Model file for the job. Use its own axes, mm. Face numbers are marked on the shaded views. A direction names the side the tool comes from. Round coordinates to 2 decimals unless told otherwise and drop trailing zeros. Loops run counter-clockwise (first coordinate to the right, second up) from the corner with the lowest first, then second, coordinate; pieces in that order, holes last. Notation, with made-up numbers: M -21.75,59 L -3.75,59 A23 ccw -3.75,84 Z; hole C -31,80 d4. An arc over 180 degrees is marked long. Use a Markdown table: item, result. Add a question column.
Q1. Tool access for the marked faces 1 and 2: list every direction of +Z, -Z, +X, -X, +Y, -Y with a clear straight run to the whole face (end or side of a thin tool).
Q2. Pin check, flat tips, straight feed: pin 1 (1 mm diameter, centred on y = 85.5, z = -4, fed in from -X); pin 2 (6 mm diameter, centred on x = 1, z = -2.5, fed in from -Y); pin 3 (1.5 mm diameter, centred on x = 14, y = 87.5, fed in from +Z); pin 4 (5 mm diameter, centred on x = -5, y = 43, fed in from -Z). Stop position of each tip, or through.
Q3. Cut at B-B (z = 0). Give the cut face in (x, y).
Q4. Cut at C-C (y = 109.5). Give the cut face in (x, z), plus the area to 3 significant figures.
Q5. Probe line 1 (Y direction, x = 8, z = 9); line 2 (X direction, y = 116, z = 1); line 3 (X direction, y = 85.5, z = 6.5). List the from-to ranges inside material, lowest first. Write a range as from..to.
Q6. Cut at A-A (x = 0). Give the cut face in (y, z), plus the area to 3 significant figures.
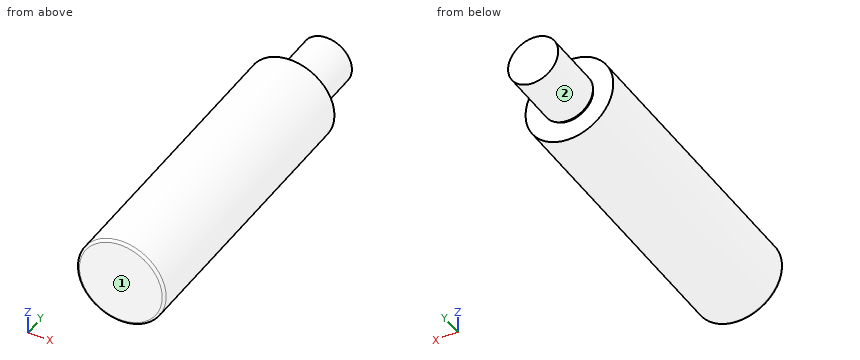
from build123d import *

# Parameters (mm, degrees)
SKETCH1_R           = 17.5
BOSS_EXTRUDE1_DEPTH = 142
SKETCH2_OUTSIDE_W   = 67.076
SKETCH2_OUTSIDE_H   = 67.076
SKETCH2_OUTSIDE_R   = 10
CUT_EXTRUDE1_DEPTH  = 25
SKETCH3_OUTSIDE_W   = 67.076
SKETCH3_OUTSIDE_H   = 67.076
SKETCH3_OUTSIDE_R   = 9.5
CUT_EXTRUDE2_DEPTH  = 1
FILLET1_R           = 1


with BuildPart() as part:
    # Sketch1 → Boss-Extrude1 (new body)
    with BuildSketch(Plane(origin=(0, 0, 0), x_dir=(1, 0, 0), z_dir=(0, 1, 0))):
        Circle(SKETCH1_R)
    extrude(amount=BOSS_EXTRUDE1_DEPTH)

    # Sketch2 outside → Cut-Extrude1 (cut)
    with BuildSketch(Plane(origin=(0, 142, 0), x_dir=(1, 0, 0), z_dir=(0, 1, 0))):
        Rectangle(SKETCH2_OUTSIDE_W, SKETCH2_OUTSIDE_H)
        Circle(SKETCH2_OUTSIDE_R, mode=Mode.SUBTRACT)
    extrude(amount=-CUT_EXTRUDE1_DEPTH, mode=Mode.SUBTRACT)

    # Sketch3 outside → Cut-Extrude2 (cut)
    with BuildSketch(Plane(origin=(0, 117, 0), x_dir=(1, 0, 0), z_dir=(0, 1, 0))):
        Rectangle(SKETCH3_OUTSIDE_W, SKETCH3_OUTSIDE_H)
        Circle(SKETCH3_OUTSIDE_R, mode=Mode.SUBTRACT)
    extrude(amount=CUT_EXTRUDE2_DEPTH, mode=Mode.SUBTRACT)

    # Fillet1
    fillet1_edges = [part.edges().sort_by_distance(p)[0] for p in [
        (-17.5, 0, 0),
    ]]
    fillet(fillet1_edges, radius=FILLET1_R)


solid = part.part
Checked values:
| question | item | result |
|---|---|---|
| 1 | face 1 | +Z, -Z, +X, -X, -Y |
| 1 | face 2 | +Y |
| 2 | pin 1 | stops at x = -17.15 |
| 2 | pin 2 | stops at y = 0 |
| 2 | pin 3 | stops at z = 11.43 |
| 2 | pin 4 | stops at z = -17.32 |
| 3 | outline | M -17.5,1 A1 ccw -16.5,0 L 16.5,0 A1 ccw 17.5,1 L 17.5,117 L 9.5,117 L 9.5,118 L 10,118 L 10,142 L -10,142 L -10,118 L -9.5,118 L -9.5,117 L -17.5,117 Z |
| 4 | outline | C 0,0 d35 |
| 4 | area | 962 mm^2 |
| 5 | line 1 | y = 0..117 |
| 5 | line 2 | x = -17.47..17.47 |
| 5 | line 3 | x = -16.25..16.25 |
| 6 | outline | M 0,-16.5 A1 ccw 1,-17.5 L 117,-17.5 L 117,-9.5 L 118,-9.5 L 118,-10 L 142,-10 L 142,10 L 118,10 L 118,9.5 L 117,9.5 L 117,17.5 L 1,17.5 A1 ccw 0,16.5 Z |
| 6 | area | 4,590 mm^2 |
